The listing builds one solid part. Answer for the finished solid, in the listing's coordinates (mm). Face numbers are marked on the shaded views. A direction names the side the tool comes from. Coordinates: 2 decimals unless noted, no trailing zeros. Loops run counter-clockwise (first coordinate to the right, second up) from the corner with the lowest first, then second, coordinate; pieces in that order, holes last. Notation, with made-up numbers: (52, 53) -> (70, 53) arc R16 cw to (70, 66) -> close; hole circle Ø6 at (85.25, 17.25). An arc over 180 degrees is marked (long way). Answer in a Markdown table with one row per item.
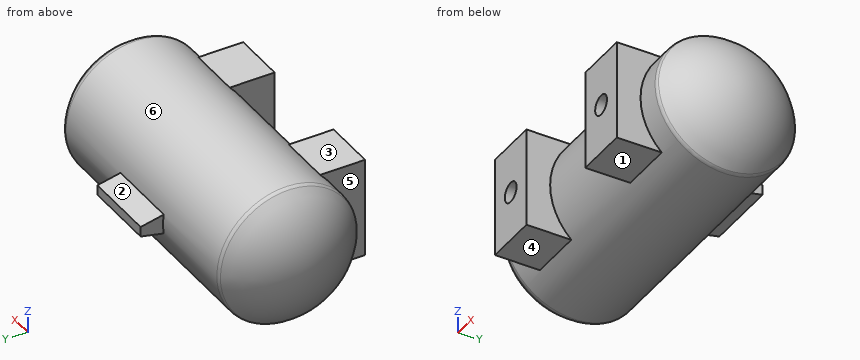
```python
from build123d import *

# Parameters (mm, degrees)
SKETCH_3_W          = 8
SKETCH_3_H          = 15
EXTRUDE_1_DEPTH     = 14
SKETCH_4_R          = 1.5
CUT_EXTRUDE_1_DEPTH = 10
FILLET_1_R          = 1
EXTRUDE_2_DEPTH     = 5.5


with BuildPart() as part:
    # ｽｹｯﾁ1 → 回転2 (revolve)
    with BuildSketch(Plane.XY):
        with BuildLine():
            Line((-19.5, 10.435516279), (19.5, 10.435516279))
            ThreePointArc((19.5, 10.435516279), (23.540844472, 5.898092912), (25, 0))
            Line((25, 0), (-25, 0))
            ThreePointArc((-25, 0), (-23.540844472, 5.898092912), (-19.5, 10.435516279))
        make_face()
    revolve(axis=Axis((-19.5, 0, 0), (1, 0, 0)))

    # ｽｹｯﾁ3 → ﾎﾞｽ - 押し出し1 (add)
    with BuildSketch(Plane(origin=(0, 0, 0), x_dir=(1, 0, 0), z_dir=(0, 1, 0))):
        with Locations((-11.5, 0)):
            Rectangle(SKETCH_3_W, SKETCH_3_H)
        with Locations((11.5, 0)):
            Rectangle(SKETCH_3_W, SKETCH_3_H)
    extrude(amount=-EXTRUDE_1_DEPTH)

    # ｽｹｯﾁ4 → ｶｯﾄ - 押し出し1 (cut)
    with BuildSketch(Plane(origin=(0, -14, 0), x_dir=(-1, 0, 0), z_dir=(0, -1, 0))):
        with Locations(Location((-11.5, 0, 0), (0, 0, 90))):
            Circle(SKETCH_4_R)
        with Locations(Location((11.5, 0, 0), (0, 0, 90))):
            Circle(SKETCH_4_R)
    extrude(amount=-CUT_EXTRUDE_1_DEPTH, mode=Mode.SUBTRACT)

    # ﾌｨﾚｯﾄ1
    fillet_1_edges = [part.edges().sort_by_distance(p)[0] for p in [
        (-19.5, -10.435516279, 0),
        (19.5, -10.435516279, 0),
    ]]
    fillet(fillet_1_edges, radius=FILLET_1_R)

    # ｽｹｯﾁ5 → ﾎﾞｽ - 押し出し2 (add, symmetric)
    with BuildSketch(Plane(origin=(0, 0, 0), x_dir=(0, 0, -1), z_dir=(1, 0, 0))):
        Polygon((-1.6, 9.8), (1.6, 9.8), (0.75, 13.8), (-0.75, 13.8), align=None)
    extrude(amount=EXTRUDE_2_DEPTH, both=True)


solid = part.part
```
Item 1: A tool of negligible diameter and unlimited length cuts with its end or side. For the marked faces 1, 2 and 3, from which of +Z, -Z, +X, -X, +Y, -Y can it reach the whole face along a straight path? Write none if from no direction.
Findings below:
| item | result |
|---|---|
| face 1 | -Z, +X, -X, -Y |
| face 2 | +Z, +X, -X, +Y |
| face 3 | +Z, +X, -X, -Y |
Item 2: A cutting plane is placed at B-B, the plane y = -9.75. Count the separate pieces of the cut face and the enclosed holes in it, plus the area to 3 significant figures.
Findings below:
| item | result |
|---|---|
| separate pieces | 1 |
| enclosed holes | 2 |
| area | 406 mm2 |
Item 3: A cutting plane is placed at A-A, the plane x = -11.5. Determine the outline of the cut face in (y, z), plus the area to 3 significant figures.
Findings below:
| item | result |
|---|---|
| outline | (-14, -7.5) -> (-7.26, -7.5) arc R10.44 ccw (long way) to (-7.26, 7.5) -> (-14, 7.5) -> (-14, 1.5) -> (-4, 1.5) -> (-4, -1.5) -> (-14, -1.5) -> close |
| area | 380 mm2 |
Item 4: Flat-ended cylindrical pins translate along their axes: pin 1 Ø2 at (y, z) = (-12, 1.5) entering from +X; pin 2 Ø2 at (y, z) = (-10.5, -1) entering from -X; pin 3 Ø2.5 at (y, z) = (12.5, 0) entering from -X. Find the tip coordinate at first contact, or state that the pin passes through.
Findings below:
| item | result |
|---|---|
| pin 1 | stops at x = 15.5 |
| pin 2 | stops at x = -20.65 |
| pin 3 | stops at x = -5.5 |
Item 5: A cutting plane is placed at C-C, the plane x = 1. Determine the outline of the cut face in (y, z), plus the area to 3 significant figures.
Findings below:
| item | result |
|---|---|
| outline | (10.33, -1.49) -> (13.8, -0.75) -> (13.8, 0.75) -> (10.33, 1.49) arc R10.44 ccw (long way) to start |
| area | 350 mm2 |
Item 6: Determine the mould class of the marked faces 4, 5 and 6 for opening direction X: +X half, -X half, draft (parallel to the pull), parting line (faces both ways), or undercut.
Findings below:
| item | result |
|---|---|
| face 4 | draft |
| face 5 | -X half |
| face 6 | undercut |
Item 7: Find the intervals of material crossed by probe 1 along X at (y, z) = (-11.5, 0); probe 2 along Y at (x, z) = (-18, -0.5); probe 3 along Y at (x, z) = (2.5, 0), in increasing order.
Findings below:
| item | result |
|---|---|
| probe 1 | x = -15.5 to -13, -10 to -7.5, 7.5 to 10, 13 to 15.5 |
| probe 2 | y = -10.42 to 10.42 |
| probe 3 | y = -10.44 to 13.8 |
Item 8: A cutting plane is placed at D-D, the plane x = 12.5. Determine the outline of the cut face in (y, z).
Findings below:
| item | result |
|---|---|
| outline | (-14, -7.5) -> (-7.26, -7.5) arc R10.44 ccw (long way) to (-7.26, 7.5) -> (-14, 7.5) -> (-14, 1.12) -> (-4, 1.12) -> (-4, -1.12) -> (-14, -1.12) -> close |
